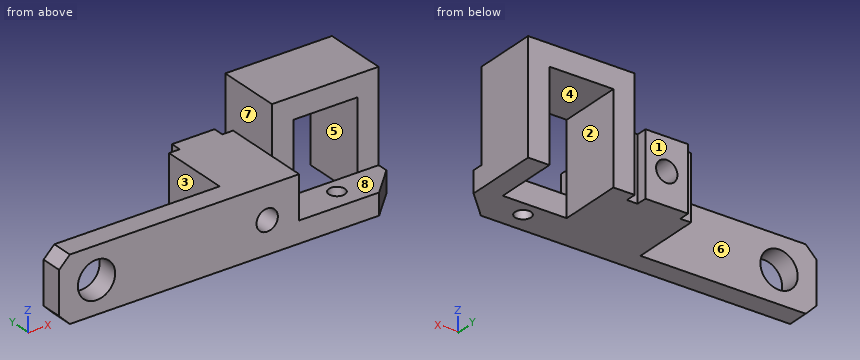
```python
from build123d import *

# Parameters (mm, degrees)
SKETCH1_W           = 33
SKETCH1_H           = 12
SKETCH1_R           = 3.5
BOSS_EXTRUDE1_DEPTH = 4
SKETCH1_4_W         = 2
SKETCH1_4_H         = 12
BOSS_EXTRUDE2_DEPTH = 17
SKETCH1_5_W         = 8
SKETCH1_5_H         = 12
SKETCH1_5_R         = 2
BOSS_EXTRUDE3_DEPTH = 19
SKETCH1_6_W         = 20
SKETCH1_6_H         = 4
BOSS_EXTRUDE4_DEPTH = 7
BOSS_EXTRUDE5_DEPTH = 12
CHAMFER1_SIZE       = 2
SKETCH3_R           = 1.5
CUT_EXTRUDE1_DEPTH  = 50.560569004


with BuildPart() as part:
    # Sketch1 → Boss-Extrude1 (new body)
    with BuildSketch(Plane(origin=(0, 0, 0), x_dir=(1, 0, 0), z_dir=(0, 1, 0))):
        with Locations((-6, 0)):
            Rectangle(SKETCH1_W, SKETCH1_H)
        with Locations(Location((-15.5, 0, 0), (0, 0, 270))):
            Circle(SKETCH1_R, mode=Mode.SUBTRACT)
    extrude(amount=BOSS_EXTRUDE1_DEPTH)

    # Sketch1<4> → Boss-Extrude2 (add)
    with BuildSketch(Plane(origin=(0, 0, 0), x_dir=(1, 0, 0), z_dir=(0, 1, 0))):
        with Locations((11.5, 0)):
            Rectangle(SKETCH1_4_W, SKETCH1_4_H)
        Polygon((22.5, 6), (20.5, 6), (20.5, -6), (22.5, -6), (22.5, 2), align=None)
    extrude(amount=BOSS_EXTRUDE2_DEPTH)


with BuildPart() as boss_extrude2_piece_1:
    # of the separate pieces the step leaves, piece 1, a body of its own (boss_extrude2_pieces)
    add(part.part.solids().sort_by_distance((-22.5, 0, -6))[0])



with BuildPart() as boss_extrude2_piece_2:
    # of the separate pieces the step leaves, piece 2, a body of its own (boss_extrude2_pieces)
    add(part.part.solids().sort_by_distance((20.5, 0, 6))[0])


with BuildPart() as boss_extrude2_piece_1_1:
    add(boss_extrude2_piece_1.part)

    add(boss_extrude2_piece_2.part)  # Boss-Extrude3 merges Boss-Extrude2 piece 2
    # Sketch1<5> → Boss-Extrude3 (add)
    with BuildSketch(Plane(origin=(0, 0, 0), x_dir=(1, 0, 0), z_dir=(0, 1, 0))):
        with Locations((16.5, 0)):
            Rectangle(SKETCH1_5_W, SKETCH1_5_H)
        with Locations(Location((16.5, 0, 0), (0, 0, 270))):
            Circle(SKETCH1_5_R, mode=Mode.SUBTRACT)
    extrude(amount=BOSS_EXTRUDE3_DEPTH)

    # Sketch1<6> → Boss-Extrude4 (add)
    with BuildSketch(Plane(origin=(0, 0, 0), x_dir=(1, 0, 0), z_dir=(0, 1, 0))):
        with Locations((32.5, 4)):
            Rectangle(SKETCH1_6_W, SKETCH1_6_H)
    extrude(amount=BOSS_EXTRUDE4_DEPTH)

    # Sketch2 → Boss-Extrude5 (add)
    with BuildSketch(Plane(origin=(0, 7, 0), x_dir=(1, 0, 0), z_dir=(0, 1, 0))):
        Polygon((22.5, 6), (26.5, 6), (26.5, 2), (26.5, -11), (38.5, -11), (38.5, 2), (38.5, 6), (42.5, 6), (42.5, -15), (22.5, -15), align=None)
    extrude(amount=BOSS_EXTRUDE5_DEPTH)

    # Chamfer1
    chamfer1_edges = [boss_extrude2_piece_1_1.edges().sort_by_distance(p)[0] for p in [
        (-22.5, 2, 6),
        (-22.5, 2, -6),
    ]]
    chamfer(chamfer1_edges, length=CHAMFER1_SIZE)

    # Sketch3 → Cut-Extrude1 (cut, through all)
    with BuildSketch(Plane.XY.offset(-2)):
        with Locations((32.5, 4)):
            Circle(SKETCH3_R)
        Polygon((42.5, 0), (42.5, 5), (37.5, 0), align=None)
    extrude(amount=-CUT_EXTRUDE1_DEPTH, mode=Mode.SUBTRACT)


solid = boss_extrude2_piece_1_1.part
```
The model under review builds one solid part; all positions refer to its coordinate system, in mm. Face numbers are marked on the shaded views. A direction names the side the tool comes from. Round coordinates to 2 decimals unless told otherwise and drop trailing zeros. Write each loop counter-clockwise with the first axis right and the second up, starting at its lowest first coordinate (ties: lowest second). Pieces come first, ordered by that corner, then holes.
(1) Insertion check: pin 1 (3 mm diameter, centred on y = 8.5, z = 8, fed in from -X); pin 2 (6 mm diameter, centred on x = 31.5, y = 13.5, fed in from -Z); pin 3 (3.5 mm diameter, centred on x = -0.5, z = -0.5, fed in from +Y); pin 4 (1.5 mm diameter, centred on y = 4.5, z = 9, fed in from +X). Each pin has a flat end and moves straight along its axis. Give the tip position at first contact, or say it passes through.
(2) Mouldability with a two-part tool opening along X and no side actions: class the marked faces 1, 2, 3 and 4 as +X half, -X half, draft (parallel to the pull), parting line (faces both ways), or undercut.
(3) We need section A-A on z = 8.5. Give the boundary of the cut face in (x, y).
(4) We need section C-C on y = 15. Give the boundary of the cut face in (x, z).
(5) We need section B-B on x = 16.5. Give the boundary of the cut face in (y, z).
(6) Machinability: for the marked faces 5, 6, 7 and 8, which of the approach directions +Z, -Z, +X, -X, +Y, -Y give a long, thin tool a straight path to every point of the face, cutting with its end or side? Answer none if there is none.
(7) Wall thickness on L1, parallel to X at y = 1.7, z = 0; L2, parallel to X at y = 13, z = 0; L3, parallel to X at y = 9.5, z = 10: over which ranges is each line inside the solid? List them lowest first.
(8) We need section D-D on z = 0. Give the boundary of the cut face in (x, y), and give its area (3 significant figures).
Findings below:
1. pin 1: stops at x = 22.5
1. pin 2: stops at z = 11
1. pin 3: stops at y = 4
1. pin 4: passes through
2. face 1: draft
2. face 2: undercut
2. face 3: -X half
2. face 4: undercut
3. outline: (22.5, 7) - (26.5, 7) - (26.5, 19) - (22.5, 19) - close; (38.5, 7) - (42.5, 7) - (42.5, 19) - (38.5, 19) - close
4. outline: (10.5, -6) - (26.5, -6) - (26.5, 11) - (38.5, 11) - (38.5, -6) - (42.5, -6) - (42.5, 15) - (22.5, 15) - (22.5, 6) - (10.5, 6) - close; hole circle Ø4 at (16.5, 0)
5. outline: (0, -6) - (19, -6) - (19, -2) - (0, -2) - close; (0, 2) - (19, 2) - (19, 6) - (0, 6) - close
6. face 5: -Z, +Y
6. face 6: +Z, -Z, -X, +Y
6. face 7: +Z, +Y
6. face 8: +Z, +X, -Y
7. L1: x = -22.5 to -19, -12 to 14.5, 18.5 to 22.5
7. L2: x = 10.5 to 14.5, 18.5 to 26.5, 38.5 to 42.5
7. L3: x = 22.5 to 26.5, 38.5 to 42.5
8. outline: (-22.5, 0) - (-19, 0) - (-19, 4) - (-22.5, 4) - close; (-12, 0) - (14.5, 0) - (14.5, 19) - (12.5, 19) - (12.5, 17) - (10.5, 17) - (10.5, 4) - (-12, 4) - close; (18.5, 0) - (22.5, 0) - (22.5, 7) - (26.5, 7) - (26.5, 19) - (22.5, 19) - (22.5, 17) - (20.5, 17) - (20.5, 19) - (18.5, 19) - close; (38.5, 7) - (42.5, 7) - (42.5, 19) - (38.5, 19) - close
8. area: 344 mm2
